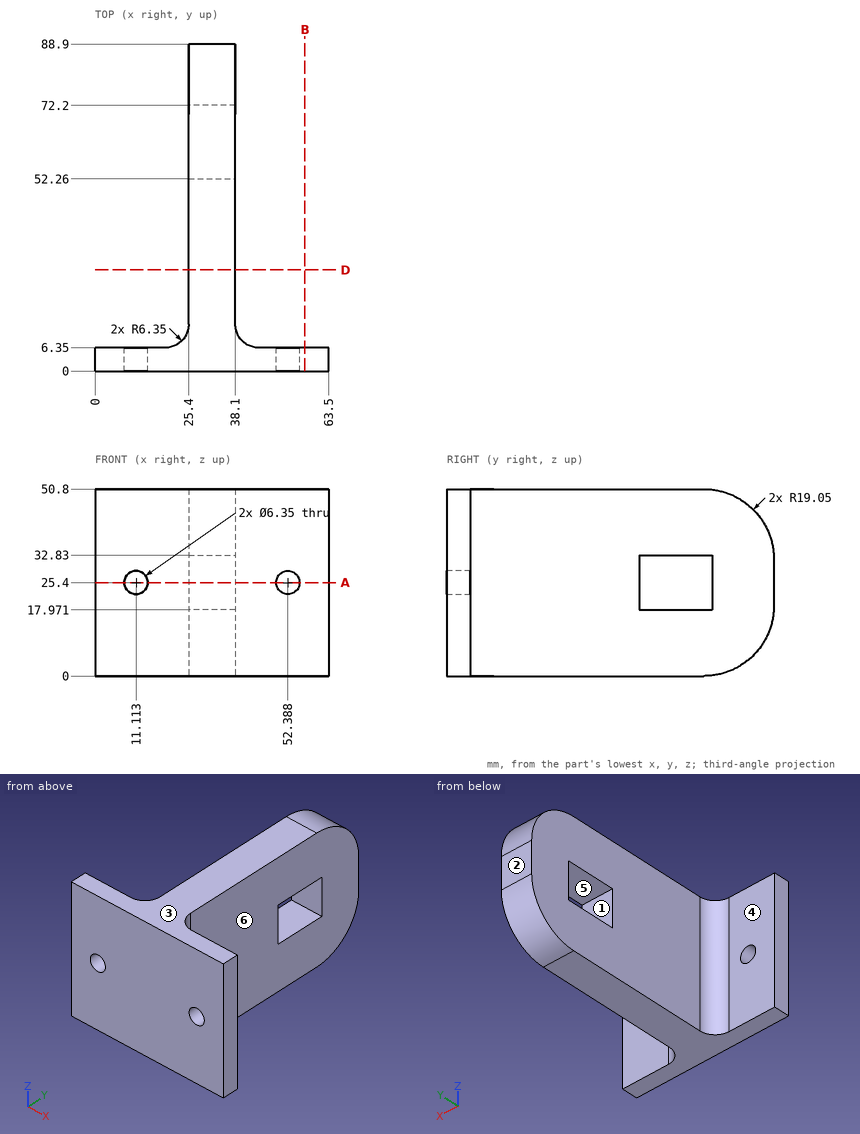
Verification items for this drawing (mm, ordinates from the low corner). A direction names the side the tool comes from. Coordinates: 2 decimals unless noted, no trailing zeros. Write each loop counter-clockwise with the first axis right and the second up, starting at its lowest first coordinate (ties: lowest second). Pieces come first, ordered by that corner, then holes. Notation, with made-up numbers: M 32,44.25 L 40,44.25 A10 ccw 40,58.25 Z; hole C -5,47.5 d4. An arc over 180 degrees is marked long. Use CSV: the item, a comma, the result in double quotes.
Q1. Section check B-B, the plane x = 57. Enter the section's corners in (y, z).
Computed values:
outline,"M 0,0 L 6.35,0 L 6.35,50.8 L 0,50.8 Z"
Q2. Section check A-A, the plane z = 25.4. Enter the section's corners in (x, y).
Computed values:
outline,"M 0,0 L 7.94,0 L 7.94,6.35 L 0,6.35 Z; M 14.29,0 L 49.21,0 L 49.21,6.35 L 44.45,6.35 A6.35 cw 38.1,12.7 L 38.1,52.26 L 25.4,52.26 L 25.4,12.7 A6.35 cw 19.05,6.35 L 14.29,6.35 Z; M 25.4,72.2 L 38.1,72.2 L 38.1,88.9 L 25.4,88.9 Z; M 55.56,0 L 63.5,0 L 63.5,6.35 L 55.56,6.35 Z"
Q3. Thickness scan on line 1 along X through (y, z) = (2, 25.4); line 2 along Y through (x, z) = (27.5, 23.5); line 3 along X through (y, z) = (19.5, 12). Record the ranges inside material, lowest first. Write a range as [from, to].
Computed values:
line 1,"[0, 7.94], [14.29, 49.21], [55.56, 63.5]"
line 2,"[0, 52.26], [72.2, 88.9]"
line 3,"[25.4, 38.1]"
Q4. Set-up check for the marked faces 4, 5 and 6: record each of +Z, -Z, +X, -X, +Y, -Y from which the full face is reachable in a straight line by a thin tool's end or side.
Computed values:
face 4,"+Z, -Z, -X, +Y"
face 5,"+X, -X"
face 6,"+Z, -Z, +X, +Y"
Q5. Mould release check, pull along Y, two halves, no side actions. Record for the marked faces 1, 2 and 3: pulls with the +Y half, pulls with the -Y half, needs draft (parallel to the pull), parting line crosses it, or undercut.
Computed values:
face 1,"undercut"
face 2,"pulls with the +Y half"
face 3,"needs draft"
Q6. Section check D-D, the plane y = 27.5. Enter the section's corners in (x, z), and give its area (3 significant figures).
Computed values:
outline,"M 25.4,0 L 38.1,0 L 38.1,50.8 L 25.4,50.8 Z"
area,"645 mm²"
Q7. Go/stop test with flat-tipped pins: P1, Ø9.5, axis at x = 54, z = 35.5, coming from the +Y side; P2, Ø12, axis at y = 56.5, z = 9.5, coming from the -X side; P3, Ø6, axis at x = 21, z = 37.5, coming from the +Y side. Record where each tip stops, or that it passes through.
Computed values:
P1,"y = 6.35"
P2,"x = 25.4"
P3,"y = 8.72"
